```python
from build123d import *

# Parameters (mm, degrees)
F_6_40_TAPPED_HOLE1_REACH  = 74.325
F_6_40_TAPPED_HOLE1_BORE_R = 1.4351
CIRPATTERN1_COUNT          = 4
FILLET1_R                  = 0.635
FILLET2_R                  = 25.4


with BuildPart() as part:
    # Sketch2 → Revolve1 (revolve)
    with BuildSketch(Plane.XY, mode=Mode.PRIVATE) as revolve1_sk:
        Polygon((22.0472, -22.4282), (22.0472, -0.0762), (27.1907, -0.0762), (27.1907, 10.922), (28.8925, 10.922), (28.8925, -0.0762), (23.8252, -32.512), (21.7932, -32.512), (21.7932, -22.4282), align=None)
    revolve(revolve1_sk.sketch.rotate(Axis((0, -34.5451, 0), (0, 1, 0)), 90), axis=Axis((0, -34.5451, 0), (0, 1, 0)))

    # #6-40 Tapped Hole1 bore → #6-40 Tapped Hole1 (cut, up to next)
    with BuildSketch(Plane.XY.offset(28.8925), mode=Mode.PRIVATE) as f_6_40_tapped_hole1_sk1:
        with Locations((0, -4.318)):
            Circle(F_6_40_TAPPED_HOLE1_BORE_R)
    f_6_40_tapped_hole1_tool1 = extrude(f_6_40_tapped_hole1_sk1.sketch, amount=-F_6_40_TAPPED_HOLE1_REACH, mode=Mode.PRIVATE) & part.part
    f_6_40_tapped_hole1 = f_6_40_tapped_hole1_tool1.solids().sort_by_distance((0, -4.318, 28.8925))[0]
    add(f_6_40_tapped_hole1, mode=Mode.SUBTRACT)

    # CirPattern1: #6-40 Tapped Hole1 ×4 about axis
    cirpattern1_axis = Axis((0, -34.5451, 0), (0, -1, 0))
    for i in range(1, CIRPATTERN1_COUNT):
        add(f_6_40_tapped_hole1.rotate(cirpattern1_axis, i * 360 / CIRPATTERN1_COUNT), mode=Mode.SUBTRACT)

    # Fillet1
    fillet1_edges = [part.edges().sort_by_distance(p)[0] for p in [
        (0, -32.512, 23.8252),
    ]]
    fillet(fillet1_edges, radius=FILLET1_R)

    # Fillet2
    fillet2_edges = [part.edges().sort_by_distance(p)[0] for p in [
        (0, -0.0762, 28.8925),
    ]]
    fillet(fillet2_edges, radius=FILLET2_R)


solid = part.part
```
The model under review builds one solid part; all positions refer to its coordinate system, in mm. A direction names the side the tool comes from. Give positions to 0.01 mm unless a question says otherwise; leave off trailing zeros. Write each loop counter-clockwise with the first axis right and the second up, starting at its lowest first coordinate (ties: lowest second). Pieces come first, ordered by that corner, then holes. Notation, with made-up numbers: M 88,39.25 L 92,39.25 A12 cw 92,44.25 Z; hole C 4.25,24 d9. An arc over 180 degrees is marked long. Write each question's results on one line, items separated by ' | '. Start each with the question number.
1. For probe 1 along Z at (x, y) = (-19, 0); probe 2 along X at (y, z) = (-3, -17.5); probe 3 along Z at (x, y) = (-1.5, -26), list the stretches that pass through material, from the lowest coordinate up. Write a range as [from, to].
2. For faces 4 (the cylindrical face through (28.205, 6.346, 6.263)), 5 (the cylindrical face through (24.12, 5.5, -12.55)), list the 3-axis set-ups (+Z, -Z, +X, -X, +Y, -Y) from which the entire face can be reached by the end or side of a thin tool; tool diameter is ignored.
3. We need section A-A (y = 4). Write out the cut boundary in (x, z) (1 decimal), and give its area (3 significant figures).
4. We need section D-D (y = -13). Write out the cut boundary in (x, z).
5. Mouldability with a two-part tool opening along X and no side actions: class faces 1 (the cylindrical face through (-25.272, -2.895, -0.187)), 2 (the flat face through (-22.3, -0.076, -0.1)), 3 (the conical face through (-7.72, -20.54, -24.51)) as released by +X, released by -X, zero draft, split by the parting line, or undercut.
6. Insertion check: pin 1 Ø3 at (y, z) = (-17, -10.5) entering from -X; pin 2 Ø1.5 at (x, y) = (11, -16) entering from -Z; pin 3 Ø4.5 at (x, y) = (0, -4.318) entering from +Z; pin 4 Ø1.7 at (x, y) = (0, -4.318) entering from -Z. Each pin has a flat end and moves straight along its axis. Give the tip position at first contact, or say it passes through.
7. We need section B-B (z = 0.5). Count the separate pieces of the cut face and the enclosed holes in it, and give its area (3 significant figures).
Results found:
1) probe 1: z = [-21.67, -19.45], [19.45, 21.67] | probe 2: x = [-22.41, -13.41], [13.41, 22.41] | probe 3: z = [-24.8, -21.74], [21.74, 24.8]
2) face 4: +Y, -Y | face 5: +Y
3) outline: C 0,0 d57.8; hole C 0,0 d54.4 | area: 300 mm^2
4) outline: C 0,0 d53.75; hole C 0,0 d44.09
5) face 1: zero draft | face 2: undercut | face 3: split by the parting line
6) pin 1: stops at x = -24.71 | pin 2: stops at z = -24.36 | pin 3: stops at z = 28.58 | pin 4: passes through
7) separate pieces: 4 | enclosed holes: 0 | area: 289 mm^2
